CAD build for the part. Positions are in the model's coordinates, mm. A direction names the side the tool comes from. Give positions to 0.01 mm unless a question says otherwise; leave off trailing zeros. Write each loop counter-clockwise with the first axis right and the second up, starting at its lowest first coordinate (ties: lowest second). Pieces come first, ordered by that corner, then holes. Notation, with made-up numbers: (61, -28) -> (92, -28) arc R20 cw to (92, 6) -> close; hole circle Ø2 at (75, 33.25). An arc over 180 degrees is marked (long way). Use one line per item in the form item = value. Start each with the question number.
from build123d import *

# Parameters (mm, degrees)
SKETCH1_R           = 2.05
SKETCH1_R_2         = 15.875
SKETCH1_R_3         = 11.1125
BOSS_EXTRUDE1_DEPTH = 1.5875
FILLET1_R           = 1.5875


with BuildPart() as part:
    # Sketch1 → Boss-Extrude1 (new body)
    with BuildSketch(Plane.XY):
        Polygon((165.1, 12.7), (139.7, 12.7), (139.7, -12.7), (165.1, -12.7), (165.1, 3.4e-08), align=None)
        with Locations((146.05, -6.35)):
            Circle(SKETCH1_R, mode=Mode.SUBTRACT)
        with Locations((158.75, 6.35)):
            Circle(SKETCH1_R, mode=Mode.SUBTRACT)
        with BuildLine():
            Line((177.490243902, 15.487804878), (165.1, 12.7))
            Line((165.1, 12.7), (165.1, 3.4e-08))
            ThreePointArc((165.1, 3.4e-08), (168.578707661, 9.917033893), (177.490243902, 15.487804878))
        make_face()
        with Locations((180.975, 0)):
            Circle(SKETCH1_R_2)
        with Locations((180.975, 0)):
            Circle(SKETCH1_R_3, mode=Mode.SUBTRACT)
        with BuildLine():
            ThreePointArc((177.490243902, -15.487804878), (168.57870764, -9.917033867), (165.1, 3.4e-08))
            Line((165.1, 3.4e-08), (165.1, -12.7))
            Line((165.1, -12.7), (177.490243902, -15.487804878))
        make_face()
    extrude(amount=BOSS_EXTRUDE1_DEPTH)

    # Fillet1
    fillet1_edges = [part.edges().sort_by_distance(p)[0] for p in [
        (165.1, 12.7, 0.79375),
        (165.1, -12.7, 0.79375),
        (139.7, -12.7, 0.79375),
        (139.7, 12.7, 0.79375),
    ]]
    fillet(fillet1_edges, radius=FILLET1_R)


solid = part.part
1) Wall check: line 1 along Y through (x, z) = (146.05, 0.6); line 2 along Y through (x, z) = (158.75, 0.45); line 3 along Y through (x, z) = (164.5, 1.5). Give the ranges that are in metal, low to high. Write a range as from..to.
2) Cut at D-D (y = -6.35). Give the cut face in (x, z).
3) Cut at C-C (z = 1.3). State how many separate pieces and enclosed holes the cut face has, and give its area (3 significant figures).
4) Cut at B-B (x = 146.05). Give the cut face in (y, z).
5) Two-plate mould, pull along Y, no slides. Class faces 4 (the face through (144.423, -7.597, 0.783)), 5 (the face through (140.15, -12.22, 0.8)), 6 (the face through (196.845, -0.398, 0.783)): released by +Y, released by -Y, zero draft, split by the parting line, or undercut.
6) 3-axis set-ups, long thin cutter, end or side, ignore diameter. For faces 1 (the face through (153, -12.7, 1)), 2 (the face through (191.574, 3.338, 0.783)), 3 (the face through (153, 12.7, 1)): which of +Z, -Z, +X, -X, +Y, -Y reach the whole face in a straight line?
7) Cut at A-A (y = 0). Give the cut face in (x, z), and give its area (3 significant figures).
Final values:
q1.line_1 = -12.7..-8.4, -4.3..12.7
q1.line_2 = -12.7..4.3, 8.4..12.7
q1.line_3 = -12.7..12.7
q2.outline = (139.7, 0) -> (144, 0) -> (144, 1.59) -> (139.7, 1.59) -> close; (148.1, 0) -> (171.86, 0) -> (171.86, 1.59) -> (148.1, 1.59) -> close; (190.09, 0) -> (195.52, 0) -> (195.52, 1.59) -> (190.09, 1.59) -> close
q3.separate_pieces = 1
q3.enclosed_holes = 3
q3.area = 1,080 mm^2
q4.outline = (-12.7, 0) -> (-8.4, 0) -> (-8.4, 1.59) -> (-12.7, 1.59) -> close; (-4.3, 0) -> (12.7, 0) -> (12.7, 1.59) -> (-4.3, 1.59) -> close
q5.face_4 = undercut
q5.face_5 = released by -Y
q5.face_6 = split by the parting line
q6.face_1 = +Z, -Z, -X, -Y
q6.face_2 = +Z, -Z
q6.face_3 = +Z, -Z, -X, +Y
q7.outline = (139.7, 0) -> (169.86, 0) -> (169.86, 1.59) -> (139.7, 1.59) -> close; (192.09, 0) -> (196.85, 0) -> (196.85, 1.59) -> (192.09, 1.59) -> close
q7.area = 55.4 mm^2
